Here's how the part is built. I have some questions about the finished solid (model axes, mm). A direction names the side the tool comes from. Round coordinates to 2 decimals unless told otherwise and drop trailing zeros. Write each loop counter-clockwise with the first axis right and the second up, starting at its lowest first coordinate (ties: lowest second). Pieces come first, ordered by that corner, then holes. Notation, with made-up numbers: (81, 6) -> (129, 6) arc R29 cw to (129, 32) -> close; hole circle Ø4 at (43, -32). An arc over 180 degrees is marked (long way). Put each result on its own line as item: value. Start each with the question number.
1) I want a section at C-C, the plane y = 33.5. List the corners of the cut face in (x, z) for me, then the cut area to 3 significant figures.
2) Which directions (+Z, -Z, +X, -X, +Y, -Y) give clear straight access to the entire face, cutting with the end or side of a thin tool? Please do faces 4 (the flat face through (203.5, 123, 2)), 5 (the cylindrical face through (170.639, 122.745, 1.972)), 6 (the flat face through (0, 69, 2)).
3) If I drill on line 1 along X through (y, z) = (132.5, 0.9); line 2 along X through (y, z) = (40, 0.85); line 3 along X through (y, z) = (68, 1.5), over which ranges is the centre line in solid material (lowest first)? Write a range as [from, to].
4) Will this pin go through, and if not, where does the flat tip stop? P1, Ø2, axis at y = 111, z = 0.5, coming from the +X side.
5) We'd pull the mould along X, two halves only. Please class faces 1 (the flat face through (213, 57, 2)), 2 (the flat face through (75, 30, 2)), 3 (the flat face through (100, 140, 2)): released by +X, released by -X, zero draft, split by the parting line, or undercut.
6) I want a section at A-A, the plane y = 81. List the corners of the cut face in (x, z) for me, then the cut area to 3 significant figures.
7) I want a section at B-B, the plane z = 2.9. Give the number of separate pieces and of enclosed holes in the cut face, then the cut area to 3 significant figures.
from build123d import *

# Parameters (mm, degrees)
SKETCH_1_W          = 140
SKETCH_1_H          = 148
EXTRUDE_1_DEPTH     = 4
HOLE_WIZARD_M4_1_D  = 4.5
HOLE_WIZARD_M3_2_D  = 3.4
SKETCH_9_W          = 65
SKETCH_9_H          = 140
EXTRUDE_3_DEPTH     = 4
HOLE_WIZARD_M2_1_D  = 2.4
SKETCH_13_W         = 9.5
SKETCH_13_H         = 29
CUT_EXTRUDE_1_DEPTH = 5
HOLE_WIZARD_M3_1_D  = 3.4
FILLET_12_R         = 7.5
FILLET_11_R         = 3


with BuildPart() as part:
    # ｽｹｯﾁ1 → ﾎﾞｽ - 押し出し1 (new body)
    with BuildSketch(Plane(origin=(0, 0, 0), x_dir=(0, 1, 0), z_dir=(0, 0, 1))):
        with Locations((70, -74)):
            Rectangle(SKETCH_1_W, SKETCH_1_H)
        Polygon((110, -124), (30, -124), (30, -74), (30, -24), (110, -24), align=None, mode=Mode.SUBTRACT)
    extrude(amount=EXTRUDE_1_DEPTH)

    # M4 すきま穴1 (through all)
    with Locations(Plane.XY.offset(4)):
        with Locations((7.5, 132.5), (140.5, 132.5), (7.5, 7.5), (140.5, 7.5)):
            Hole(HOLE_WIZARD_M4_1_D / 2)

    # M3 すきま穴2 (through all)
    with Locations(Plane.XY.offset(4)):
        with Locations((44, 117.5), (104, 117.5), (104, 22.5), (44, 22.5)):
            Hole(HOLE_WIZARD_M3_2_D / 2)

    # ｽｹｯﾁ9 → ﾎﾞｽ - 押し出し3 (add)
    with BuildSketch(Plane.XY.offset(4)):
        with Locations((180.5, 70)):
            Rectangle(SKETCH_9_W, SKETCH_9_H)
    extrude(amount=-EXTRUDE_3_DEPTH)

    # M2 すきま穴1 (through all)
    with Locations(Plane.XY.offset(4)):
        with Locations((203, 10), (154, 68), (203, 68), (154, 10)):
            Hole(HOLE_WIZARD_M2_1_D / 2)

    # ｽｹｯﾁ13 → ｶｯﾄ - 押し出し1 (cut, through all)
    with BuildSketch(Plane.XY.offset(4)):
        Polygon((168.5, 125), (188.5, 125), (188.5, 103), (196, 103), (196, 15), (161, 15), (161, 103), (168.5, 103), align=None)
        with Locations((208.25, 125.5)):
            Rectangle(SKETCH_13_W, SKETCH_13_H)
    extrude(amount=-CUT_EXTRUDE_1_DEPTH, mode=Mode.SUBTRACT)

    # M3 すきま穴1 (through all)
    with Locations(Plane.XY.offset(4)):
        with Locations((163.5, 125), (193.5, 125)):
            Hole(HOLE_WIZARD_M3_1_D / 2)

    # ﾌｨﾚｯﾄ12
    fillet_12_edges = [part.edges().sort_by_distance(p)[0] for p in [
        (168.5, 125, 2),
        (188.5, 125, 2),
        (196, 15, 2),
        (161, 15, 2),
        (203.5, 140, 2),
        (24, 30, 2),
        (124, 30, 2),
        (124, 110, 2),
        (24, 110, 2),
        (213, 0, 2),
        (0, 0, 2),
        (0, 140, 2),
    ]]
    fillet(fillet_12_edges, radius=FILLET_12_R)

    # ﾌｨﾚｯﾄ11
    fillet_11_edges = [part.edges().sort_by_distance(p)[0] for p in [
        (168.5, 103, 2),
        (188.5, 103, 2),
        (196, 103, 2),
        (161, 103, 2),
        (213, 111, 2),
        (203.5, 111, 2),
    ]]
    fillet(fillet_11_edges, radius=FILLET_11_R)


solid = part.part
Findings:
1. outline: (0, 0) -> (25.16, 0) -> (25.16, 4) -> (0, 4) -> close; (122.84, 0) -> (161, 0) -> (161, 4) -> (122.84, 4) -> close; (196, 0) -> (213, 0) -> (213, 4) -> (196, 4) -> close
1. area: 321 mm2
2. face 4: +Z, -Z, +X, +Y
2. face 5: +Z, -Z
2. face 6: +Z, -Z, -X, +Y, -Y
3. line 1: x = [0, 5.25], [9.75, 138.25], [142.75, 203.5]
3. line 2: x = [0, 24], [124, 161], [196, 213]
3. line 3: x = [0, 24], [124, 152.8], [155.2, 161], [196, 201.8], [204.2, 213]
4. P1: stops at x = 212.24
5. face 1: released by +X
5. face 2: undercut
5. face 3: zero draft
6. outline: (0, 0) -> (24, 0) -> (24, 4) -> (0, 4) -> close; (124, 0) -> (161, 0) -> (161, 4) -> (124, 4) -> close; (196, 0) -> (213, 0) -> (213, 4) -> (196, 4) -> close
6. area: 312 mm2
7. separate pieces: 1
7. enclosed holes: 16
7. area: 17,900 mm2
